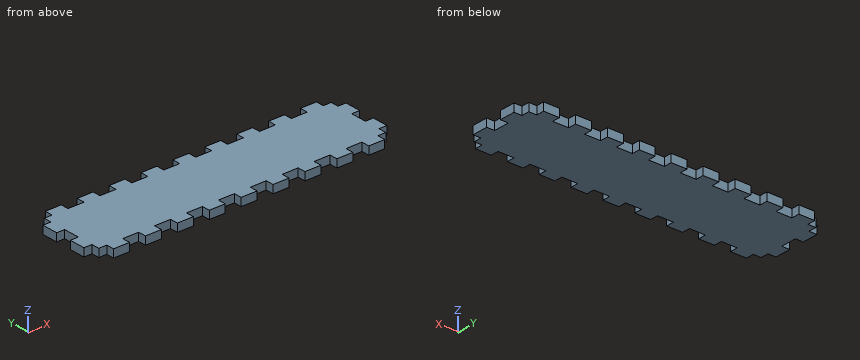
from build123d import *

# Parameters (mm, degrees)
SKETCH2_W           = 241.3
SKETCH2_H           = 63.5
BOSS_EXTRUDE1_DEPTH = 6.35
SKETCH3_W           = 6.35
SKETCH3_H           = 12.7
CUT_EXTRUDE1_DEPTH  = 7.35
LPATTERN1_COUNT     = 3
LPATTERN1_PITCH     = 25.4
SKETCH4_W           = 12.7
SKETCH4_H           = 6.35
CUT_EXTRUDE2_DEPTH  = 7.35
LPATTERN2_COUNT     = 10
LPATTERN2_PITCH     = 25.4


with BuildPart() as part:
    # Sketch2 → Boss-Extrude1 (new body)
    with BuildSketch(Plane.XY):
        with Locations((120.65, 31.75)):
            Rectangle(SKETCH2_W, SKETCH2_H)
    extrude(amount=BOSS_EXTRUDE1_DEPTH)

    # Sketch3 → Cut-Extrude1 (cut, through all)
    with BuildSketch(Plane.XY.offset(6.35)):
        with Locations((3.175, 57.15)):
            Rectangle(SKETCH3_W, SKETCH3_H)
        with Locations((238.125, 57.15)):
            Rectangle(SKETCH3_W, SKETCH3_H)
    cut_extrude1 = extrude(amount=-CUT_EXTRUDE1_DEPTH, mode=Mode.SUBTRACT)

    # LPattern1: Cut-Extrude1 ×3
    with Locations(*[(0, -i * LPATTERN1_PITCH, 0) for i in range(1, LPATTERN1_COUNT)]):
        add(cut_extrude1, mode=Mode.SUBTRACT)

    # Sketch4 → Cut-Extrude2 (cut, through all)
    with BuildSketch(Plane.XY.offset(6.35)):
        with Locations((6.35, 60.325)):
            Rectangle(SKETCH4_W, SKETCH4_H)
        with Locations((6.35, 3.175)):
            Rectangle(SKETCH4_W, SKETCH4_H)
    cut_extrude2 = extrude(amount=-CUT_EXTRUDE2_DEPTH, mode=Mode.SUBTRACT)

    # LPattern2: Cut-Extrude2 ×10
    with Locations(*[(i * LPATTERN2_PITCH, 0, 0) for i in range(1, LPATTERN2_COUNT)]):
        add(cut_extrude2, mode=Mode.SUBTRACT)


solid = part.part
Input: part model. Units: mm. Frame: model coordinates. Coordinates: 2 decimals unless noted, no trailing zeros. Loops run counter-clockwise (first coordinate to the right, second up) from the corner with the lowest first, then second, coordinate; pieces in that order, holes last. Notation, with made-up numbers: (-26, 14) -> (-4, 14) arc R24 cw to (-4, 35) -> close; hole circle Ø11 at (17.25, 42.25). An arc over 180 degrees is marked (long way). Write each question's results on one line, items separated by ' | '. Start each with the question number.
Q1. Ray query, line 1 (X direction, y = 30.5, z = 6.25); line 2 (Y direction, x = 164.5, z = 6.25). Return the intervals inside material, ascending. Write a range as from..to.
Q2. Section A-A, the plane y = 59.5. State how many separate pieces and enclosed holes the cut face has, plus the area to 3 significant figures.
Q3. Section C-C, the plane x = 155. Return the cut outline in (y, z).
Q4. Section B-B, the plane y = 28. Return the cut outline in (x, z), plus the area to 3 significant figures.
Q5. Pin query (flat end, axial travel): pin 1 (3 mm diameter, centred on y = 33.5, z = 4.5, fed in from -X); pin 2 (3 mm diameter, centred on y = 3, z = 3, fed in from -X); pin 3 (1.9 mm diameter, centred on x = 82.5, z = 4, fed in from +Y). Return the tip coordinate at first contact, or that it passes through.
Found:
1) line 1: 6.35..234.95 | line 2: 6.35..57.15
2) separate pieces: 9 | enclosed holes: 0 | area: 726 mm2
3) outline: (6.35, 0) -> (57.15, 0) -> (57.15, 6.35) -> (6.35, 6.35) -> close
4) outline: (6.35, 0) -> (234.95, 0) -> (234.95, 6.35) -> (6.35, 6.35) -> close | area: 1,450 mm2
5) pin 1: x = 6.35 | pin 2: x = 12.7 | pin 3: y = 57.15
